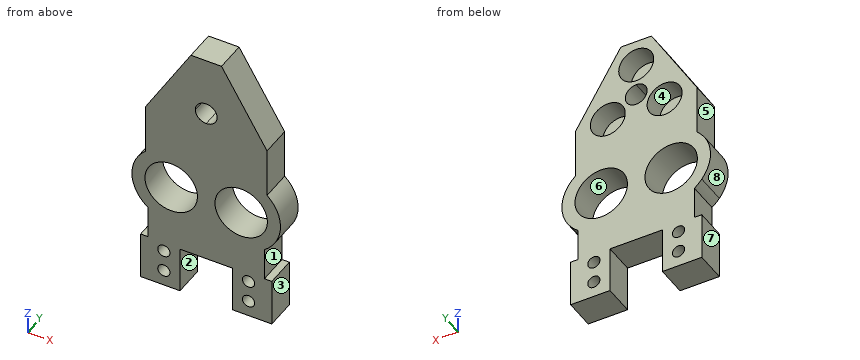
Autodesk Inventor part; units mm, degrees
ref_plane "YZ Plane" through (0, 0, 0) normal (1, 0, 0) x (0, 1, 0)
ref_plane "XZ Plane" through (0, 0, 0) normal (0, 1, 0) x (-1, 0, 0)
ref_plane "XY Plane" through (0, 0, 0) normal (0, 0, 1) x (1, 0, 0)
ref_plane "Work Plane8" through (-7.4556, -16.4352, 24.63) normal (0, 1, 0) x (0, 0, -1)
sketch "Sketch12" plane through (-7.4556, -16.4352, 24.63) normal (0, 1, 0) x (0, 0, -1)
  circle A0 centre (31.71, -8) radius 6 construction
  circle A1 centre (31.71, 8) radius 6 construction
  line L0 (59.1648, 4.9103) -> (72.1552, 12.4103) construction
  arc A2 (80.66, 7.5) -> (72.1552, 12.4103) centre (70.66, 0) ccw construction
  line L1 (80.66, 7.5) -> (80.66, -7.5) construction
  arc A3 (72.1552, -12.4103) -> (80.66, -7.5) centre (70.66, 0) ccw construction
  line L2 (72.1552, -12.4103) -> (59.1648, -4.9103) construction
  arc A4 (59.1648, 4.9103) -> (59.1648, -4.9103) centre (70.66, 0) ccw construction
  line L3 (57.3131, 5.945) -> (46.6951, 5.945) construction
  line L4 (46.6951, 5.945) -> (46.6951, -5.9961)
  line L5 (46.6951, -5.9961) -> (57.3131, -5.9961)
  line L6 (57.3131, -5.9961) -> (57.3131, -15)
  line L7 (57.3131, -15) -> (85.66, -15) construction
  line L8 (85.66, -15) -> (85.66, 15) construction
  line L9 (85.66, 15) -> (57.3131, 15) construction
  line L10 (57.3131, 15) -> (57.3131, 5.945) construction
  line L11 (46.6951, -6.3061) -> (57.3131, -6.3061)
  line L12 (3.89, -16.97) -> (37.83, -16.97)
  line L13 (41.63, -16.87) -> (45.71, -16.87)
  line L14 (55.66, -15) -> (46.2855, -13.3689)
  line L15 (55.66, -15) -> (105.1976, -15) construction
  line L16 (46.6951, 0) -> (46.6951, -6.3061)
  arc A5 (24.9318, -13.9208) -> (37.3669, -15) centre (31.71, -8) ccw
  line L17 (24.9318, -13.9208) -> (13.5861, -13.9208)
  line L18 (-3.79, -3.4952) -> (-3.79, 3.4952)
  line L19 (-3.79, 0) -> (-3.79, 0)
  line L20 (-3.79, 0) -> (-3.79, -3.4952)
  line L21 (-3.79, -3.4952) -> (13.5861, -13.9208)
  line L22 (46.6951, 0) -> (-3.79, 0)
  line L23 (57.3131, -6.3061) -> (57.3131, -15)
  line L24 (57.3131, -15) -> (37.3669, -15)
  line L25 (-3.79, -8.16) -> (-3.79, 8.16)
  line L26 (19.46, 16.4952) -> (10.1021, 16.4952)
  line L27 (19.46, -16.4952) -> (19.46, 16.4952)
  line L28 (10.1021, -16.4952) -> (19.46, -16.4952)
  line L29 (10.1021, 16.4952) -> (-3.79, 8.16)
  line L30 (-3.79, -8.16) -> (10.1021, -16.4952)
  circle A6 centre (9.71, 0) radius 1.75
  point P0 (24.63, -7.4556)
  point P1 (11.21, -12.4952)
  point P2 (19.46, 12.4952)
  point P3 (19.46, -12.4952)
extrude "Extrusion11" add sketch "Sketch12" along normal blind 7 contours L4 L16 L11 L6 L24 A5 L12 L17 L27 L22 | L5 L6 L11 L16 | L27 L17 L21 L18 L22 A6 | A6 L22 | L12 A5 picked at (9.6397, -0.5791)
sketch "Sketch13" plane through (-7.4556, -9.4352, 24.63) normal (0, 1, 0) x (1, 0, 0)
  circle A0 centre (8, 31.71) radius 6
  circle A1 centre (8, 31.71) radius 6.1
  circle A2 centre (9.6825, 53.6267) radius 1.4
  circle A3 centre (9.6825, 48.6267) radius 1.4
  circle A4 centre (0, 9.71) radius 2.5
  point P0 (7.4556, 24.63)
  dimension "d68" = 12.2
extrude "Extrusion12" cut sketch "Sketch13" against normal through all contours A0 | A2 | A3 | A4
sketch "Sketch16" plane through (-7.4556, -9.4352, 24.63) normal (0, 1, 0) x (1, 0, 0)
  line L0 (13.9208, 13.5861) -> (13.9208, 24.9318)
  arc A0 (13.9208, 24.9318) -> (15, 37.3669) centre (8, 31.71) ccw
  line L1 (5.9961, 46.6951) -> (0, 46.6951)
  line L2 (13.8689, 40.3869) -> (13.8689, 45.71)
  line L3 (15, 39.0186) -> (13.3086, 39.0186)
  line L4 (13.3086, 39.0186) -> (13.3086, 46.45)
  line L5 (13.3086, 46.45) -> (15, 46.45)
  line L6 (15, 46.45) -> (15, 39.0186)
  arc A1 (15, 37.3669) -> (13.3086, 39.0186) centre (7.8235, 31.71) ccw
  line L7 (13.3086, 46.45) -> (15, 48.1414)
  line L8 (15, 37.3669) -> (15, 57.3131)
  line L9 (13.3086, 46.45) -> (15.7006, 46.45) construction
  line L10 (15, 48.1414) -> (15, 46.45)
  line L11 (15, 39.0186) -> (15, 37.3669)
  line L12 (0, 7.21) -> (0, -3.79)
  line L13 (0, -3.79) -> (3.4952, -3.79)
  line L14 (3.4952, -3.79) -> (13.9208, 13.5861)
  line L15 (15, 37.3669) -> (15, 57.3131)
  line L16 (15, 57.3131) -> (5.9961, 57.3131)
  line L17 (5.9961, 57.3131) -> (5.9961, 46.6951)
  arc A2 (0, 7.21) -> (0, 12.21) centre (0, 9.71) ccw
  line L18 (0, 46.6951) -> (0, 12.21)
  point P0 (7.4556, 24.63)
  dimension "d80" = 45
extrude "Extrusion15" cut sketch "Sketch16" against normal through all contours A1 L3 L8 | L4 L5 L6 L3
mirror "Mirror3" about plane through (-7.4556, -16.4352, -22.0651) normal (-1, 0, 0) of "Extrusion11", "Extrusion12", "Extrusion15"
sketch "Sketch17" plane through (-7.4556, -9.4352, 24.63) normal (0, 1, 0) x (1, 0, 0)
  circle A0 centre (6.4952, 13.46) radius 4
  circle A1 centre (0, 2.21) radius 4
  circle A2 centre (-6.4952, 13.46) radius 4
  point P0 (7.4556, 24.63)
extrude "Extrusion16" cut sketch "Sketch17" against normal blind 5
properties part number "30_Cube_Z_Focus_MGN_NEMA_slide_part2"
The model under review builds one solid part; all positions refer to its coordinate system, in mm. Face numbers are marked on the shaded views. A direction names the side the tool comes from. Give positions to 0.01 mm unless a question says otherwise; leave off trailing zeros. Loops run counter-clockwise (first coordinate to the right, second up) from the corner with the lowest first, then second, coordinate; pieces in that order, holes last. Notation, with made-up numbers: (-22, -15) -> (29, -15) arc R24 cw to (29, 12) -> close; hole circle Ø5 at (50.5, -17). An arc over 180 degrees is marked (long way). Put each result on its own line as item: value. Start each with the question number.
1. Clearance check with flat-ended pins moving along their axes: P1, Ø3.5, axis at y = -12.5, z = 4.5, coming from the -X side; P2, Ø7, axis at x = -0.96, z = 11.17, coming from the +Y side; P3, Ø4, axis at y = -14, z = -17.5, coming from the -X side; P4, Ø11, axis at x = 0.54, z = -7.08, coming from the -Y side. State where each tip first meets the part, or that it passes through.
2. We need section A-A on z = -27. State the section outline as (x, y) points, then the cut area to 3 significant figures.
3. We need section C-C on y = -12. State how many separate pieces and enclosed holes the cut face has, then the cut area to 3 significant figures.
4. Mouldability with a two-part tool opening along Z and no side actions: class the marked faces 6, 7 and 8 as released by +Z, released by -Z, zero draft, split by the parting line, or undercut.
5. We need section B-B on x = 4.5. State the section outline as (y, z) points.
6. Wall thickness on probe 1 along X at (y, z) = (-11.25, -7.08); probe 2 along X at (y, z) = (-11, -26); probe 3 along X at (y, z) = (-11.5, 11): over which ranges is each line inside the solid? List them lowest first.
7. We need section D-D on z = 22.42. State the section outline as (x, y) points, then the cut area to 3 significant figures.
8. For the marked faces 1, 2, 3, 4 and 5, list the 3-axis set-ups (+Z, -Z, +X, -X, +Y, -Y) from which the entire face can be reached by the end or side of a thin tool; tool diameter is ignored.
Determined:
1. P1: x = -21.38
1. P2: y = -14.44
1. P3: x = -20.76
1. P4: through
2. outline: (-22.46, -16.44) -> (-13.45, -16.44) -> (-13.45, -9.44) -> (-22.46, -9.44) -> close; (-1.46, -16.44) -> (7.54, -16.44) -> (7.54, -9.44) -> (-1.46, -9.44) -> close
2. area: 126 mm^2
3. separate pieces: 1
3. enclosed holes: 10
3. area: 1,040 mm^2
4. face 6: undercut
4. face 7: zero draft
4. face 8: split by the parting line
5. outline: (-16.44, -32.68) -> (-9.44, -32.68) -> (-9.44, -11.59) -> (-16.44, -11.59) -> close; (-16.44, -2.57) -> (-9.44, -2.57) -> (-9.44, 14.32) -> (-16.44, 14.32) -> close
6. probe 1: -24.46 to -21.46, -9.46 to -5.46, 6.54 to 9.54
6. probe 2: -22.46 to -13.45, -1.46 to 7.54
6. probe 3: -21.38 to -17.95, -9.95 to -4.96, 3.04 to 6.47
7. outline: (-14.55, -16.44) -> (-0.36, -16.44) -> (-0.36, -9.44) -> (-3.46, -9.44) -> (-3.46, -14.44) -> (-11.46, -14.44) -> (-11.46, -9.44) -> (-14.55, -9.44) -> close
7. area: 59.3 mm^2
8. face 1: +X, +Y, -Y
8. face 2: -Z, +Y, -Y
8. face 3: -Z, +X, +Y, -Y
8. face 4: +Y
8. face 5: +Z, -X, +Y, -Y
